The model under review builds one solid part; all positions refer to its coordinate system, in mm. Coordinates: 2 decimals unless noted, no trailing zeros. Write each loop counter-clockwise with the first axis right and the second up, starting at its lowest first coordinate (ties: lowest second). Pieces come first, ordered by that corner, then holes.
1) For line 1 (Z direction, x = 1, y = 181.5); line 2 (Z direction, x = -1.75, y = 260.5); line 3 (Y direction, x = -1, z = 1612), list the stretches that pass through material, from the lowest coordinate up.
2) Add section A-A, the plane x = 3.25. State the section outline as (y, z) points, then the cut area to 3 significant figures.
3) For P1, Ø1.5, axis at x = -0.5, y = 100, coming from the +Z side; P2, Ø6, axis at x = 1, y = 334, coming from the -Z side; P3, Ø3, axis at x = 4, y = 317, coming from the -Z side, all flat-tipped, find the tip position at first contact; note any pin that passes through.
4) Add section B-B, the plane y = 60.5. State the section outline as (x, z) points, then the cut area to 3 significant figures.
from build123d import *

# Parameters (mm, degrees)
SKETCH_1_R      = 5
EXTRUDE_1_DEPTH = 1780
SKETCH_2_R      = 5
EXTRUDE_2_DEPTH = 452


with BuildPart() as part:
    # 草图1 → 凸台-拉伸1 (new body)
    with BuildSketch(Plane.XY):
        Circle(SKETCH_1_R)
    extrude(amount=EXTRUDE_1_DEPTH)

    # 草图2 → 凸台-拉伸2 (add)
    with BuildSketch(Plane(origin=(0, 0, 0), x_dir=(1, 0, 0), z_dir=(0, 1, 0))):
        with Locations((0, -300)):
            Circle(SKETCH_2_R)
        with Locations((0, -1480)):
            Circle(SKETCH_2_R)
    extrude(amount=EXTRUDE_2_DEPTH)


solid = part.part
Geometry results:
1. line 1: z = 295.1 to 304.9, 1475.1 to 1484.9
1. line 2: z = 295.32 to 304.68, 1475.32 to 1484.68
1. line 3: y = -4.9 to 4.9
2. outline: (-3.8, 0) - (3.8, 0) - (3.8, 296.2) - (452, 296.2) - (452, 303.8) - (3.8, 303.8) - (3.8, 1476.2) - (452, 1476.2) - (452, 1483.8) - (3.8, 1483.8) - (3.8, 1780) - (-3.8, 1780) - close
2. area: 20,300 mm2
3. P1: stops at z = 1485
3. P2: stops at z = 295
3. P3: stops at z = 295.67
4. outline: circle Ø10 at (0, 300); circle Ø10 at (0, 1480)
4. area: 157 mm2
